from build123d import *

# Parameters (mm, degrees)
SKIZZE1_W                                      = 68
SKIZZE1_H                                      = 55
AUFSATZ_LINEAR_AUSTRAGEN1_DEPTH                = 78
SKIZZE2_W                                      = 58
SKIZZE2_H                                      = 68
SCHNITT_LINEAR_AUSTRAGEN1_DEPTH                = 118.187883333
SKIZZE3_R                                      = 5
AUFSATZ_LINEAR_AUSTRAGEN2_DEPTH                = 10
STIRNSENKUNG_START                             = 73
STIRNSENKUNG_LANGLOCH_F_R_M6_SENKSCHRAUB_DEPTH = 3.3
STIRNSENKUNG_START_2                           = 76.3
STIRNSENKUNG_LANGLOCH_F_R_M6_SENKSCH_3_DEPTH   = 1.7
SCHNITT_LINEAR_AUSTRAGEN2_DEPTH                = 5


# Read off the part's stored shape, not the designer's step: Stirnsenkung Langloch für M6 Senkschraube (Kopf Button)1
with BuildPart() as part:
    # Skizze1 → Aufsatz-Linear austragen1 (new body)
    with BuildSketch(Plane.XY):
        with Locations((-34, 27.5)):
            Rectangle(SKIZZE1_W, SKIZZE1_H)
    extrude(amount=AUFSATZ_LINEAR_AUSTRAGEN1_DEPTH)

    # Skizze2 → Schnitt-Linear austragen1 (cut, through all)
    with BuildSketch(Plane(origin=(0, 55, 0), x_dir=(1, 0, 0), z_dir=(0, 1, 0))):
        with Locations((-34, -39)):
            Rectangle(SKIZZE2_W, SKIZZE2_H)
    extrude(amount=-SCHNITT_LINEAR_AUSTRAGEN1_DEPTH, mode=Mode.SUBTRACT)

    # Skizze3 → Aufsatz-Linear austragen2 (add)
    with BuildSketch(Plane.XY.offset(78)):
        with Locations((-32.5, 30)):
            Circle(SKIZZE3_R)
    extrude(amount=AUFSATZ_LINEAR_AUSTRAGEN2_DEPTH)

    # Stirnsenkung Langloch f_r M6 Senksch 2 → Stirnsenkung Langloch für M6 Senkschraube (Kopf Button)1 (cut)
    with BuildSketch(Plane.XY.offset(STIRNSENKUNG_START)):
        with BuildLine():
            ThreePointArc((-12.25, 36.5), (-18, 42.25), (-23.75, 36.5))
            Line((-23.75, 36.5), (-23.75, 13.5))
            ThreePointArc((-23.75, 13.5), (-18, 7.75), (-12.25, 13.5))
            Line((-12.25, 13.5), (-12.25, 36.5))
        make_face()
    extrude(amount=STIRNSENKUNG_LANGLOCH_F_R_M6_SENKSCHRAUB_DEPTH, mode=Mode.SUBTRACT)

    # Stirnsenkung Langloch f_r M6 Senksch 3 o → Stirnsenkung Langloch f_r M6 Senksch 3 (cut)
    with BuildSketch(Plane.XY.offset(STIRNSENKUNG_START_2)):
        with BuildLine():
            ThreePointArc((-14.5, 36.5), (-18, 40), (-21.5, 36.5))
            Line((-21.5, 36.5), (-21.5, 13.5))
            ThreePointArc((-21.5, 13.5), (-18, 10), (-14.5, 13.5))
            Line((-14.5, 13.5), (-14.5, 36.5))
        make_face()
    extrude(amount=STIRNSENKUNG_LANGLOCH_F_R_M6_SENKSCH_3_DEPTH, mode=Mode.SUBTRACT)

    # Skizze15 → Schnitt-Linear austragen2 (cut)
    with BuildSketch(Plane.XZ):
        Polygon((0, 0), (-5, 8.660254038), (-63, 8.660254038), (-68, 0), align=None)
    extrude(amount=-SCHNITT_LINEAR_AUSTRAGEN2_DEPTH, mode=Mode.SUBTRACT)


solid = part.part
The model under review builds one solid part; all positions refer to its coordinate system, in mm. A direction names the side the tool comes from. Give positions to 0.01 mm unless a question says otherwise; leave off trailing zeros. Loops run counter-clockwise (first coordinate to the right, second up) from the corner with the lowest first, then second, coordinate; pieces in that order, holes last. Notation, with made-up numbers: (62, -39) -> (76, -39) arc R9 cw to (76, -33) -> close; hole circle Ø6 at (68, -12). An arc over 180 degrees is marked (long way). Write each question's results on one line, items separated by ' | '.
1) Take a section at B-B, the plane y = 20. Give the boundary of the cut face in (x, z), plus the area to 3 significant figures.
Conclusion:
outline: (-68, 0) -> (0, 0) -> (0, 78) -> (-14.5, 78) -> (-14.5, 76.3) -> (-12.25, 76.3) -> (-12.25, 73) -> (-5, 73) -> (-5, 5) -> (-63, 5) -> (-63, 73) -> (-23.75, 73) -> (-23.75, 76.3) -> (-21.5, 76.3) -> (-21.5, 78) -> (-68, 78) -> close | area: 1,310 mm^2
2) Draft analysis for pull direction Y (two halves, no side actions). For faces 1 (the face through (-34, 5, 2)), 2 (the face through (-34, 30, 5)), 3 (the face through (-18, 40, 77)), state which applies: pulls with the +Y half, pulls with the -Y half, needs draft (parallel to the pull), parting line crosses it, or undercut.
Conclusion:
face 1: pulls with the -Y half | face 2: needs draft | face 3: undercut
3) Tool access review of faces 4 (the face through (-17.87, 42.25, 74.63)), 5 (the face through (-34, 28, 73)), 6 (the face through (-2.465, 2.465, 4.27)): name each direction out of +Z, -Z, +X, -X, +Y, -Y from which nothing blocks a thin tool from reaching the whole face with its end or side.
Conclusion:
face 4: none | face 5: +Y, -Y | face 6: -Z, -Y
4) Take a section at D-D, the plane z = 79.5. Give the boundary of the cut face in (x, y).
Conclusion:
outline: circle Ø10 at (-32.5, 30)
5) Take a section at A-A, the plane z = 27. Give the boundary of the cut face in (x, y), plus the area to 3 significant figures.
Conclusion:
outline: (-68, 0) -> (-63, 0) -> (-63, 55) -> (-68, 55) -> close; (-5, 0) -> (0, 0) -> (0, 55) -> (-5, 55) -> close | area: 550 mm^2
6) Take a section at C-C, the plane x = -32.5. Give the boundary of the cut face in (y, z).
Conclusion:
outline: (0, 73) -> (55, 73) -> (55, 78) -> (35, 78) -> (35, 88) -> (25, 88) -> (25, 78) -> (0, 78) -> close; (5, 0) -> (55, 0) -> (55, 5) -> (5, 5) -> close
7) Insertion check: pin 1 Ø6 at (x, z) = (-59, 23.5) entering from -Y; pin 2 Ø16.5 at (x, y) = (-40, 14) entering from +Z; pin 3 Ø9.5 at (x, z) = (-44, 3.5) entering from -Y. Each pin has a flat end and moves straight along its axis. Give the tip position at first contact, or say it passes through.
Conclusion:
pin 1: passes through | pin 2: stops at z = 78 | pin 3: stops at y = 5
8) For line 1 along Z through (x, y) = (-46, 46); line 2 along X through (y, z) = (32, 46.5); line 3 along Z through (x, y) = (-22, 27), list the stretches that pass through material, from the lowest coordinate up. Write a range as from..to.
Conclusion:
line 1: z = 0..5, 73..78 | line 2: x = -68..-63, -5..0 | line 3: z = 0..5, 76.3..78
